from build123d import *

# Parameters (mm, degrees)
BOSS_EXTRUDE1_DEPTH = 1
SKETCH2_W           = 140
SKETCH2_H           = 50
BOSS_EXTRUDE2_DEPTH = 1
SKETCH3_W           = 151
SKETCH3_H           = 140
BOSS_EXTRUDE3_DEPTH = 1
SKETCH5_W           = 108.724422279
SKETCH5_H           = 140
BOSS_EXTRUDE4_DEPTH = 1
SKETCH6_R           = 2.5
BOSS_EXTRUDE5_DEPTH = 40


with BuildPart() as part:
    # Sketch1 → Boss-Extrude1 (new body)
    with BuildSketch(Plane.XY):
        Polygon((0, 0), (0, 50), (140, 50), (230, 111), (240, 111), (240, 61), (150, 0), align=None)
    boss_extrude1 = extrude(amount=BOSS_EXTRUDE1_DEPTH)

    # Sketch2 → Boss-Extrude2 (add)
    with BuildSketch(Plane.ZY):
        with Locations((-69, 25)):
            Rectangle(SKETCH2_W, SKETCH2_H)
    extrude(amount=BOSS_EXTRUDE2_DEPTH)

    # Mirror1: Boss-Extrude1 across plane
    add(boss_extrude1.mirror(Plane.XY.offset(-69)))

    # Sketch3 → Boss-Extrude3 (add)
    with BuildSketch(Plane.XZ):
        with Locations((74.5, -69)):
            Rectangle(SKETCH3_W, SKETCH3_H)
    extrude(amount=-BOSS_EXTRUDE3_DEPTH)

    # Sketch5 → Boss-Extrude4 (add)
    with BuildSketch(Plane(origin=(47.216817528, -69.664157009, 0), x_dir=(-0.8277808988368524, -0.5610514981005335, 0), z_dir=(0.5610514981005335, -0.8277808988368524, 0))):
        with Locations((-178.529345965, 69)):
            Rectangle(SKETCH5_W, SKETCH5_H)
    extrude(amount=-BOSS_EXTRUDE4_DEPTH)

    # Sketch6 → Boss-Extrude5 (add)
    with BuildSketch(Plane.XZ):
        with Locations(Location((4, -4, 0), (0, 0, 180))):
            Circle(SKETCH6_R)
        with Locations(Location((4, -134, 0), (0, 0, 180))):
            Circle(SKETCH6_R)
        with Locations(Location((145, -4, 0), (0, 0, 180))):
            Circle(SKETCH6_R)
        with Locations(Location((145, -134, 0), (0, 0, 180))):
            Circle(SKETCH6_R)
    extrude(amount=BOSS_EXTRUDE5_DEPTH)


solid = part.part
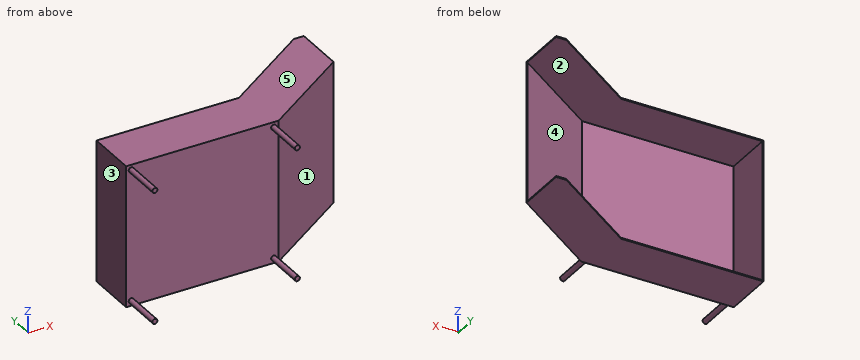
Design review of the part built by this model. Coordinates are the model's own, in mm. Face numbers are marked on the shaded views. A direction names the side the tool comes from. Coordinates: 2 decimals unless noted, no trailing zeros. Loops run counter-clockwise (first coordinate to the right, second up) from the corner with the lowest first, then second, coordinate; pieces in that order, holes last. Notation, with made-up numbers: M -29.5,63.5 L -4.5,63.5 A18 ccw -4.5,96.5 Z; hole C 61,17 d10. An arc over 180 degrees is marked long. Use one line per item in the form item = value.
(1) For line 1 along Z through (x, y) = (72.5, 20); line 2 along Y through (x, z) = (145.5, -119.5); line 3 along X through (y, z) = (38, -113), list the stretches that pass through material, from the lowest coordinate up. Write a range as from..to.
Return value:
line_1 = -139..-138, 0..1
line_2 = 0..1
line_3 = -1..0, 204.28..206.07
(2) Consider section B-B (x = 49). Write out the cut boundary in (y, z), and give its area (3 significant figures).
Return value:
outline = M 0,-139 L 50,-139 L 50,-138 L 1,-138 L 1,0 L 50,0 L 50,1 L 0,1 Z
area = 238 mm2
(3) Consider section D-D (y = 6). Write out the cut boundary in (x, z).
Return value:
outline = M -1,-139 L 158.85,-139 L 158.85,1 L -1,1 Z; hole M 0,-138 L 157.07,-138 L 157.07,0 L 0,0 Z
(4) For the marked faces 1 and 2, list the 3-axis set-ups (+Z, -Z, +X, -X, +Y, -Y) from which the entire face can be reached by the end or side of a thin tool; tool diameter is ignored.
Return value:
face_1 = +Z, -Z, +X, -Y
face_2 = +Y
(5) Draft analysis for pull direction X (two halves, no side actions). For the marked faces 3, 4 and 5, state which applies: pulls with the +X half, pulls with the -X half, needs draft (parallel to the pull), parting line crosses it, or undercut.
Return value:
face_3 = pulls with the -X half
face_4 = undercut
face_5 = needs draft
(6) Consider section A-A (y = 100.5). Write out the cut boundary in (x, z), and give its area (3 significant figures).
Return value:
outline = M 214.51,-139 L 240,-139 L 240,-138 L 214.51,-138 Z; M 214.51,0 L 240,0 L 240,1 L 214.51,1 Z
area = 51.0 mm2
(7) Consider section C-C (z = -56.5). Write out the cut boundary in (x, y).
Return value:
outline = M -1,0 L 150,0 L 240,61 L 239.44,61.83 L 149.69,1 L 0,1 L 0,50 L -1,50 Z
(8) Clearance check with flat-ended pins moving along their axes: P1, Ø24.5, axis at y = 13.5, z = -48, coming from the +X side; P2, Ø5, axis at x = 78, y = 54, coming from the -Z side; P3, Ø12, axis at x = 34, z = -39.5, coming from the +Y side. State where each tip first meets the part, or that it passes through.
Return value:
P1 = 187.99
P2 = through
P3 = 1
